Input: dimensioned drawing with shaded views. Units: mm. Origin: part minimum x, y, z. A direction names the side the tool comes from. Coordinates: 2 decimals unless noted, no trailing zeros. Order: outer loops, then holes, each group sorted by start corner. A loop starts at its lowest first (then second) coordinate and runs counter-clockwise, first axis right, second up. Notation, with made-up numbers: M -10.75,-7 L 15.25,-7 A5 ccw 15.25,2 Z; hole C 66.25,57.5 d1. An arc over 180 degrees is marked long. Use CSV: the item, a comma, the result in double quotes. Start each with the question number.
1. Section query B-B on x = 10.5. Return the cut outline in (y, z), and give its area (3 significant figures).
2. Material intervals for line 1 (Z direction, x = 27.5, y = 53); line 2 (Y direction, x = 3.5, z = 30.5); line 3 (Z direction, x = 47, y = 11), sorted ascending.
3. Set-up query: the marked faces 1 and 2. Return all of +Z, -Z, +X, -X, +Y, -Y with unobstructed straight access to the full face (end or side cutting, diameter ignored); none if empty.
4. Section query A-A on z = 23.5. Return the cut outline in (x, y).
5. Section query D-D on z = 52. Return the cut outline in (x, y), and give its area (3 significant figures).
6. Section query C-C on y = 73.5. Return the cut outline in (x, z), and give its area (3 significant figures).
7. First-contact query: P1, Ø3, axis at y = 36.5, z = 37, coming from the -X side; P2, Ø3, axis at y = 14, z = 49.5, coming from the +X side; P3, Ø2, axis at y = 22.5, z = 43, coming from the -X side. Flat tips, straight axial feed; report the tip coordinate or a pass-through.
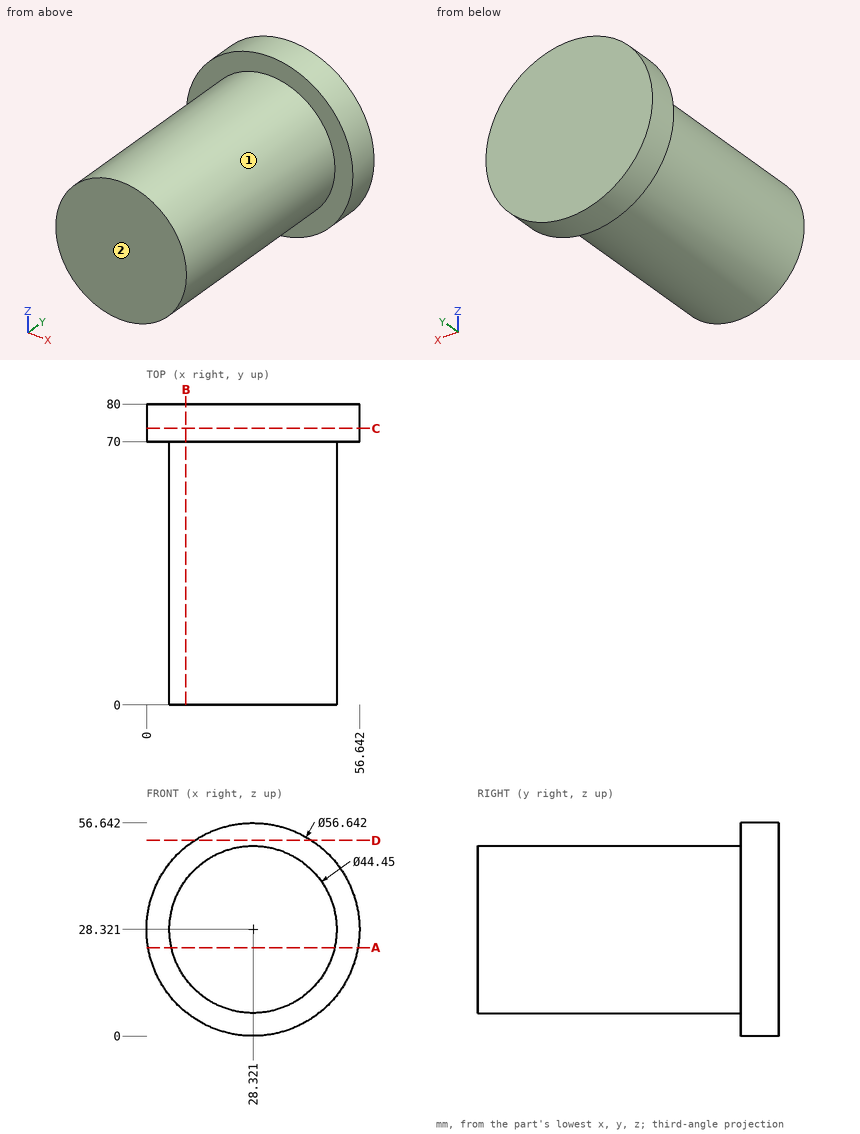
Results list:
1,outline,"M 0,15.04 L 70,15.04 L 70,6.31 L 80,6.31 L 80,50.33 L 70,50.33 L 70,41.6 L 0,41.6 Z"
1,area,"2,300 mm²"
2,line 1,"z = 6.11 to 50.53"
2,line 2,"y = 70 to 80"
2,line 3,"z = 16.28 to 40.36"
3,face 1,"-Y"
3,face 2,"+Z, -Z, +X, -X, -Y"
4,outline,"M 0.41,70 L 6.63,70 L 6.63,0 L 50.02,0 L 50.02,70 L 56.23,70 L 56.23,80 L 0.41,80 Z"
5,outline,"M 12.78,70 L 43.86,70 L 43.86,80 L 12.78,80 Z"
5,area,"311 mm²"
6,outline,"C 28.32,28.32 d56.64"
6,area,"2,520 mm²"
7,P1,"stops at x = 7.29"
7,P2,"stops at x = 38.65"
7,P3,"stops at x = 10.8"
